```python
from build123d import *

# Parameters (mm, degrees)
SKETCH1_W           = 7
SKETCH1_H           = 6
BOSS_EXTRUDE1_DEPTH = 9
SKETCH2_W           = 3
SKETCH2_H           = 1
CUT_EXTRUDE10_DEPTH = 7
CUT_EXTRUDE11_DEPTH = 1
SKETCH12_W          = 1
SKETCH12_H          = 1
CUT_EXTRUDE12_DEPTH = 5
SKETCH13_W          = 1
SKETCH13_H          = 4
CUT_EXTRUDE13_DEPTH = 7
CUT_EXTRUDE14_DEPTH = 2
SKETCH15_W          = 3
SKETCH15_H          = 2
CUT_EXTRUDE17_DEPTH = 6
SKETCH18_W          = 3
SKETCH18_H          = 1
CUT_EXTRUDE18_DEPTH = 6
SKETCH20_W          = 3
SKETCH20_H          = 3.16227766
CUT_EXTRUDE19_DEPTH = 6
SKETCH21_W          = 3
SKETCH21_H          = 4
CUT_EXTRUDE20_DEPTH = 6
SKETCH22_W          = 3
SKETCH22_H          = 1
CUT_EXTRUDE22_DEPTH = 6
SKETCH23_W          = 7
SKETCH23_H          = 2
CUT_EXTRUDE24_DEPTH = 7
SKETCH24_W          = 3
SKETCH24_H          = 1
CUT_EXTRUDE25_DEPTH = 2
SKETCH25_W          = 3
SKETCH25_H          = 1
CUT_EXTRUDE26_DEPTH = 2
SKETCH28_W          = 3
SKETCH28_H          = 2.236067977
CUT_EXTRUDE27_DEPTH = 2
SKETCH29_W          = 1
SKETCH29_H          = 2
CUT_EXTRUDE28_DEPTH = 1
SKETCH30_W          = 1
SKETCH30_H          = 2
CUT_EXTRUDE29_DEPTH = 1
SKETCH31_W          = 3
SKETCH31_H          = 2
CUT_EXTRUDE30_DEPTH = 40
CUT_EXTRUDE31_DEPTH = 3


with BuildPart() as part:
    # Sketch1 → Boss-Extrude1 (new body)
    with BuildSketch(Plane.XY):
        Rectangle(SKETCH1_W, SKETCH1_H)
    extrude(amount=BOSS_EXTRUDE1_DEPTH)

    # Sketch2 → Cut-Extrude10 (cut, through all)
    with BuildSketch(Plane(origin=(0, 3, 0), x_dir=(1, 0, 0), z_dir=(0, 1, 0))):
        with Locations((0, -8.5)):
            Rectangle(SKETCH2_W, SKETCH2_H)
    extrude(amount=-CUT_EXTRUDE10_DEPTH, mode=Mode.SUBTRACT)

    # Sketch11 → Cut-Extrude11 (cut)
    with BuildSketch(Plane(origin=(0, 0, 0), x_dir=(-1, 0, 0), z_dir=(0, 0, -1))):
        Polygon((-2.5, 3), (-3.5, 1), (-3.5, 3), align=None)
        Polygon((3.5, 3), (2.5, 3), (3.5, 1), align=None)
    extrude(amount=-CUT_EXTRUDE11_DEPTH, mode=Mode.SUBTRACT)

    # Sketch12 → Cut-Extrude12 (cut)
    with BuildSketch(Plane(origin=(0, 3, 0), x_dir=(1, 0, 0), z_dir=(0, 1, 0))):
        with Locations((3, -1.5)):
            Rectangle(SKETCH12_W, SKETCH12_H)
        with Locations((-3, -1.5)):
            Rectangle(SKETCH12_W, SKETCH12_H)
    extrude(amount=-CUT_EXTRUDE12_DEPTH, mode=Mode.SUBTRACT)

    # Sketch13 → Cut-Extrude13 (cut, through all)
    with BuildSketch(Plane(origin=(0, 3, 0), x_dir=(1, 0, 0), z_dir=(0, 1, 0))):
        with Locations((3, -4)):
            Rectangle(SKETCH13_W, SKETCH13_H)
        with Locations((-3, -4)):
            Rectangle(SKETCH13_W, SKETCH13_H)
    extrude(amount=-CUT_EXTRUDE13_DEPTH, mode=Mode.SUBTRACT)

    # Sketch14 → Cut-Extrude14 (cut)
    with BuildSketch(Plane.XY.offset(9)):
        Polygon((3.5, 3), (2.5, 3), (3.5, -2), align=None)
        Polygon((-3.5, 3), (-2.5, 3), (-3.5, -2), align=None)
    extrude(amount=-CUT_EXTRUDE14_DEPTH, mode=Mode.SUBTRACT)

    # Sketch15 → Cut-Extrude17 (cut)
    with BuildSketch(Plane.XY.offset(8)):
        with Locations((0, -2)):
            Rectangle(SKETCH15_W, SKETCH15_H)
    extrude(amount=-CUT_EXTRUDE17_DEPTH, mode=Mode.SUBTRACT)

    # Sketch18 → Cut-Extrude18 (cut)
    with BuildSketch(Plane.XY.offset(8)):
        with Locations((0, 2.5)):
            Rectangle(SKETCH18_W, SKETCH18_H)
    extrude(amount=-CUT_EXTRUDE18_DEPTH, mode=Mode.SUBTRACT)

    # Sketch20 → Cut-Extrude19 (cut)
    with BuildSketch(Plane(origin=(0, 2.3, 6.9), x_dir=(-1, 0, 0), z_dir=(0, -0.316227766, -0.948683298))):
        with Locations((0, -1.897366596)):
            Rectangle(SKETCH20_W, SKETCH20_H)
    extrude(amount=-CUT_EXTRUDE19_DEPTH, mode=Mode.SUBTRACT)

    # Sketch21 → Cut-Extrude20 (cut, through all)
    with BuildSketch(Plane(origin=(0, 2, 0), x_dir=(1, 0, 0), z_dir=(0, 1, 0))):
        with Locations((0, -4)):
            Rectangle(SKETCH21_W, SKETCH21_H)
    extrude(amount=-CUT_EXTRUDE20_DEPTH, mode=Mode.SUBTRACT)

    # Sketch22 → Cut-Extrude22 (cut)
    with BuildSketch(Plane.XY.offset(9)):
        with Locations((0, 1.5)):
            Rectangle(SKETCH22_W, SKETCH22_H)
    extrude(amount=-CUT_EXTRUDE22_DEPTH, mode=Mode.SUBTRACT)

    # Sketch23 → Cut-Extrude24 (cut)
    with BuildSketch(Plane.XY.offset(9)):
        with Locations((0, 2)):
            Rectangle(SKETCH23_W, SKETCH23_H)
    extrude(amount=-CUT_EXTRUDE24_DEPTH, mode=Mode.SUBTRACT)

    # Sketch24 → Cut-Extrude25 (cut)
    with BuildSketch(Plane.XY.offset(9)):
        Polygon((2.2, 1), (3.5, -2), (2.9, 1), align=None)
        Polygon((-2.2, 1), (-2.9, 1), (-3.5, -2), align=None)
        with Locations((0, 0.5)):
            Rectangle(SKETCH24_W, SKETCH24_H)
    extrude(amount=-CUT_EXTRUDE25_DEPTH, mode=Mode.SUBTRACT)

    # Sketch25 → Cut-Extrude26 (cut)
    with BuildSketch(Plane.XY.offset(7)):
        with Locations((0, 0.5)):
            Rectangle(SKETCH25_W, SKETCH25_H)
    extrude(amount=-CUT_EXTRUDE26_DEPTH, mode=Mode.SUBTRACT)

    # Sketch28 → Cut-Extrude27 (cut)
    with BuildSketch(Plane(origin=(0, 1, 2), x_dir=(1, 0, 0), z_dir=(0, 0.447213595, 0.894427191))):
        with Locations((0, 1.118033989)):
            Rectangle(SKETCH28_W, SKETCH28_H)
    extrude(amount=CUT_EXTRUDE27_DEPTH, mode=Mode.SUBTRACT)

    # Sketch29 → Cut-Extrude28 (cut)
    with BuildSketch(Plane(origin=(2.5, 0, 0), x_dir=(0, 0, -1), z_dir=(1, 0, 0))):
        with Locations((-1.5, 2)):
            Rectangle(SKETCH29_W, SKETCH29_H)
    extrude(amount=-CUT_EXTRUDE28_DEPTH, mode=Mode.SUBTRACT)

    # Sketch30 → Cut-Extrude29 (cut)
    with BuildSketch(Plane.ZY.offset(2.5)):
        with Locations((1.5, 2)):
            Rectangle(SKETCH30_W, SKETCH30_H)
    extrude(amount=-CUT_EXTRUDE29_DEPTH, mode=Mode.SUBTRACT)

    # Sketch31 → Cut-Extrude30 (cut)
    with BuildSketch(Plane(origin=(2.5, 0, 0), x_dir=(0, 0, -1), z_dir=(1, 0, 0))):
        with Locations((-3.5, -2)):
            Rectangle(SKETCH31_W, SKETCH31_H)
    extrude(amount=-CUT_EXTRUDE30_DEPTH, mode=Mode.SUBTRACT)

    # Sketch33 → Cut-Extrude31 (cut)
    with BuildSketch(Plane(origin=(-1.5, 0, 0), x_dir=(0, 0, -1), z_dir=(1, 0, 0))):
        Polygon((-7, 0), (-8, -1), (-8.435720839, 0.362085591), align=None)
    extrude(amount=CUT_EXTRUDE31_DEPTH, mode=Mode.SUBTRACT)


solid = part.part
```
Model file for the job. Use its own axes, mm. A direction names the side the tool comes from. Give positions to 0.01 mm unless a question says otherwise; leave off trailing zeros. Loops run counter-clockwise (first coordinate to the right, second up) from the corner with the lowest first, then second, coordinate; pieces in that order, holes last. Notation, with made-up numbers: M 29.5,84 L 70.5,84 A13 cw 70.5,90 Z; hole C 53.25,40 d2. An arc over 180 degrees is marked long. Use one line per item in the form item = value.
Item 1: Drill centre lines: L1, parallel to X at y = 0.25, z = 3.5; L2, parallel to Z at x = 3, y = -1.25; L3, parallel to X at y = -2, z = 6.25. Where is each one in solid material? Low to high.
Filled in:
L1 = -2.5 to -1.5, 1.5 to 2.5
L2 = 0 to 1, 6 to 9
L3 = -3.5 to -1.5, 1.5 to 3.5
Item 2: Slice it at D-D on y = 2. List the corners of the cut face in (x, z), and give its area (3 significant figures).
Filled in:
outline = M -3,0 L 3,0 L 3,1 L 1.5,1 L 1.5,1.5 L -1.5,1.5 L -1.5,1 L -3,1 Z
area = 7.50 mm^2
Item 3: Slice it at C-C on y = -2.5. List the corners of the cut face in (x, z).
Filled in:
outline = M -3.5,0 L 3.5,0 L 3.5,2 L -3.5,2 Z; M -3.5,6 L -2.5,6 L -2.5,5 L -1.5,5 L -1.5,9 L -3.5,9 Z; M 1.5,5 L 2.5,5 L 2.5,6 L 3.5,6 L 3.5,9 L 1.5,9 Z
Item 4: Two-plate mould, pull along Z, no slides. Class faces 1 (the flat face through (0, 2, 1.5)), 2 (the flat face through (1.5, 1.6, 1.3)), 3 (the flat face through (-1.5, -0.6, 5.5)): released by +Z, released by -Z, zero draft, split by the parting line, or undercut.
Filled in:
face_1 = released by +Z
face_2 = zero draft
face_3 = undercut
Item 5: Which spindle directions (+Z, -Z, +X, -X, +Y, -Y) get a long thin tool onto all of the face, cutting with end or side? Do faces 4 (the flat face through (0, -0.5, 7.5)), 5 (the flat face through (2, -1, 4)), 6 (the flat face through (-3, 0, 7)). Say none if no direction does.
Filled in:
face_4 = +Z, +Y
face_5 = +X, -X, -Y
face_6 = +Z, -X, +Y
Item 6: Flat gauge pins, fed straight in: pin 1 Ø2 at (x, z) = (-2, 6.5) entering from +Y; pin 2 Ø1.2 at (y, z) = (0, 4) entering from +X; pin 3 Ø3 at (y, z) = (-1, 4) entering from -X. Where does each tip first touch, or does it go through?
Filled in:
pin_1 = 1
pin_2 = 2.5
pin_3 = -2.5
Item 7: Slice it at B-B on z = 2.5. List the corners of the cut face in (x, y).
Filled in:
outline = M -2.5,-1 L -1.5,-1 L -1.5,1 L -2.5,1 Z; M 1.5,-1 L 2.5,-1 L 2.5,1 L 1.5,1 Z
Item 8: Slice it at A-A on x = 0. List the corners of the cut face in (y, z), and give its area (3 significant figures).
Filled in:
outline = M -3,0 L 3,0 L 3,1 L 1,2 L -3,2 Z; M -1,6 L 0,6 L 0,7 L -1,8 Z
area = 12.5 mm^2
